```python
from build123d import *

# Parameters (mm, degrees)
BOSS_EXTRUDE1_DEPTH = 457.2
FILLET1_R           = 0.762
FILLET2_R           = 1.524
SKETCH2_R           = 3.556
CUT_EXTRUDE1_DEPTH  = 463.273528266
SKETCH3_R           = 3.556
SKETCH3_R_2         = 3.175
CUT_EXTRUDE2_DEPTH  = 458.600012933


with BuildPart() as part:
    # Sketch1 → Boss-Extrude1 (new body)
    with BuildSketch(Plane(origin=(0, 0, 0), x_dir=(0, 0, -1), z_dir=(1, 0, 0))):
        Polygon((-50.917252699, 3.14071867), (-50.917252699, -12.73428133), (-66.792252699, -12.73428133), (-66.792252699, -11.13408133), (-52.517452699, -11.13408133), (-52.517452699, 3.14071867), align=None)
    extrude(amount=BOSS_EXTRUDE1_DEPTH)

    # Fillet1
    fillet1_edges = [part.edges().sort_by_distance(p)[0] for p in [
        (228.6, -11.13408133, 66.792252699),
        (228.6, 3.14071867, 52.517452699),
    ]]
    fillet(fillet1_edges, radius=FILLET1_R)

    # Fillet2
    fillet2_edges = [part.edges().sort_by_distance(p)[0] for p in [
        (228.6, -11.13408133, 52.517452699),
    ]]
    fillet(fillet2_edges, radius=FILLET2_R)

    # Sketch2 → Cut-Extrude1 (cut, through all)
    with BuildSketch(Plane(origin=(0, -11.13408133, 0), x_dir=(1, 0, 0), z_dir=(0, 1, 0))):
        with Locations(Location((444.5, -60.442252699, 0), (0, 0, 270))):
            Circle(SKETCH2_R)
        with Locations(Location((419.1, -60.442252699, 0), (0, 0, 270))):
            Circle(SKETCH2_R)
        with Locations(Location((12.7, -60.442252699, 0), (0, 0, 270))):
            Circle(SKETCH2_R)
        with Locations(Location((38.1, -60.442252699, 0), (0, 0, 270))):
            Circle(SKETCH2_R)
    extrude(amount=-CUT_EXTRUDE1_DEPTH, mode=Mode.SUBTRACT)

    # Sketch3 → Cut-Extrude2 (cut, through all)
    with BuildSketch(Plane.XY.offset(52.517452699)):
        with Locations((12.7, -3.20928133)):
            Circle(SKETCH3_R)
        with Locations((444.5, -3.20928133)):
            Circle(SKETCH3_R_2)
    extrude(amount=-CUT_EXTRUDE2_DEPTH, mode=Mode.SUBTRACT)


solid = part.part
```
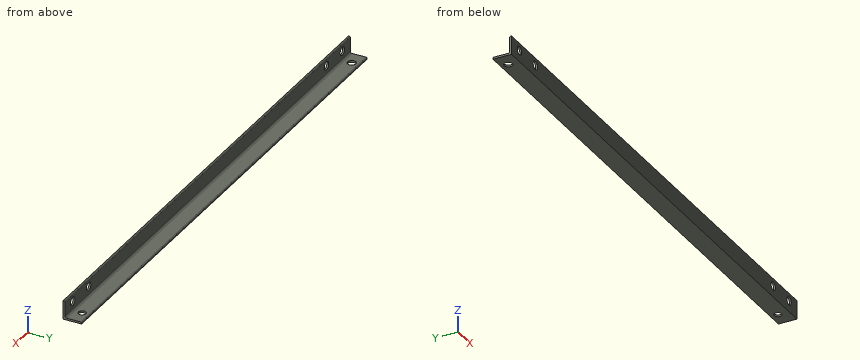
Verification items for the finished model (mm, model axes). Coordinates: 2 decimals unless noted, no trailing zeros. Loops run counter-clockwise (first coordinate to the right, second up) from the corner with the lowest first, then second, coordinate; pieces in that order, holes last. Notation, with made-up numbers: (40, 33) -> (65, 33) arc R16 cw to (65, 51) -> close; hole circle Ø8 at (84, 77). An arc over 180 degrees is marked (long way). Put each result on its own line as item: value.
1. Gauge pin test, flat ends, axial feed: P1, Ø8, axis at x = 419.1, z = 60.44, coming from the +Y side; P2, Ø1.5, axis at x = 386.5, y = -1.5, coming from the +Z side; P3, Ø5.5, axis at x = 12.7, z = 60.44, coming from the +Y side. Record the tip position at first contact, or that the pin passes through.
Result set:
P1: stops at y = -11.13
P2: stops at z = 52.52
P3: passes through
2. Thickness scan on line 1 (Z direction, x = 47, y = -7); line 2 (Y direction, x = 444.5, z = 51.3); line 3 (Y direction, x = 437, z = 61.25). Record the ranges inside material, lowest first.
Result set:
line 1: z = 50.92 to 52.52
line 2: y = -12.73 to -6.38, -0.03 to 3.14
line 3: y = -12.73 to -11.13
3. Section check A-A, the plane z = 60. Record the boundary of the cut face in (x, y).
Result set:
outline: (0, -12.73) -> (9.17, -12.73) -> (9.17, -11.13) -> (0, -11.13) -> close; (16.23, -12.73) -> (34.57, -12.73) -> (34.57, -11.13) -> (16.23, -11.13) -> close; (41.63, -12.73) -> (415.57, -12.73) -> (415.57, -11.13) -> (41.63, -11.13) -> close; (422.63, -12.73) -> (440.97, -12.73) -> (440.97, -11.13) -> (422.63, -11.13) -> close; (448.03, -12.73) -> (457.2, -12.73) -> (457.2, -11.13) -> (448.03, -11.13) -> close
4. Section check B-B, the plane x = 381.5. Record the boundary of the cut face in (y, z).
Result set:
outline: (-12.73, 50.92) -> (3.14, 50.92) -> (3.14, 51.76) arc R0.76 ccw to (2.38, 52.52) -> (-9.61, 52.52) arc R1.52 cw to (-11.13, 54.04) -> (-11.13, 66.03) arc R0.76 ccw to (-11.9, 66.79) -> (-12.73, 66.79) -> close
